The listing builds one solid part. Answer for the finished solid, in the listing's coordinates (mm). A direction names the side the tool comes from. Give positions to 0.01 mm unless a question says otherwise; leave off trailing zeros. Loops run counter-clockwise (first coordinate to the right, second up) from the corner with the lowest first, then second, coordinate; pieces in that order, holes last. Notation, with made-up numbers: (8.5, -18) - (13.5, -18) arc R21 cw to (13.5, -1) - close; hole circle Ø11 at (20, 82). An arc over 180 degrees is marked (long way). Answer as CSV lines item,"result". Start each with the question number.
1) A cutting plane is placed at D-D (z = -90.5). Determine the outline of the cut face in (x, y).
2) Flat-ended cylindrical pins translate along their axes: pin 1 (21 mm diameter, centred on x = -50.5, z = -56, fed in from +Y); pin 2 (1 mm diameter, centred on x = -27.5, z = -137, fed in from +Y). Find the tip coordinate at first contact, or state that the pin passes through.
3) For faces 1 (the face through (-50, 6, -26.65)), 2 (the face through (-49, 4, -65.65)), 3 (the face through (-3, 16, -162)), determine the directions among +Z, -Z, +X, -X, +Y, -Y from which every point of the face is accessible in a straight line to the end or side of a thin tool.
4) Find the intervals of material crossed by line 1 along X through (y, z) = (5.5, -114); line 2 along Z through (x, y) = (-57, 3.5); line 3 along X through (y, z) = (1.75, -34.5), in increasing order.
5) For a pull along Z with two mould halves and no side action, classify faces 4 (the face through (-48, 5, 0)), 5 (the face through (-92, 16, -3)), 6 (the face through (-70, 4, -111.5)) as pulls with the +Z half, pulls with the -Z half, needs draft (parallel to the pull), parting line crosses it, or undercut.
6) A cutting plane is placed at A-A (z = -40.5). Determine the outline of the cut face in (x, y), and give its area (3 significant figures).
7) A cutting plane is placed at B-B (x = -28.5). Determine the outline of the cut face in (y, z), and give its area (3 significant figures).
8) A cutting plane is placed at C-C (x = -57). Determine the outline of the cut face in (y, z).
Autodesk Inventor part; units mm, degrees
ref_plane "YZ Plane" through (0, 0, 0) normal (1, 0, 0) x (0, 1, 0)
ref_plane "XZ Plane" through (0, 0, 0) normal (0, 1, 0) x (-1, 0, 0)
ref_plane "XY Plane" through (0, 0, 0) normal (0, 0, 1) x (1, 0, 0)
sketch "草圖1" plane through (0, 0, 0) normal (0, 1, 0) x (-1, 0, 0)
  line L0 (0, 0) -> (95, 0)
  line L1 (95, 0) -> (95, -165)
  line L2 (95, -165) -> (0, -165)
  line L3 (0, -165) -> (0, 0)
  dimension "d0" = 95
  dimension "d1" = 165
extrude "擠出1" add sketch "草圖1" along normal blind 5
sketch "草圖2" plane through (0, 5, 0) normal (0, 1, 0) x (1, 0, 0)
  circle A0 centre (-3, 3) radius 1.5
  line L0 (0, 0) -> (0, 165)
  line L1 (-95, 0) -> (0, 0)
  circle A1 centre (-92, 3) radius 1.5
  line L2 (-95, 165) -> (-95, 0)
  circle A2 centre (-92, 162) radius 1.5
  line L3 (0, 165) -> (-95, 165)
  circle A3 centre (-3, 162) radius 1.5
  dimension "d4" = 3
  dimension "d5" = 3
  dimension "d6" = 3
  dimension "d7" = 3
  dimension "d8" = 3
  dimension "d9" = 3
  dimension "d10" = 3
  dimension "d11" = 3
  dimension "d12" = 3
  dimension "d13" = 3
  dimension "d14" = 3
  dimension "d15" = 3
extrude "擠出2" add sketch "草圖2" along normal blind 11 contours A0 | A1 | A2 | A3
sketch "草圖3" plane through (0, 0, 0) normal (0, -1, 0) x (1, 0, 0)
  line L0 (-25, -60.15) -> (-20, -60.15)
  line L1 (-20, -60.15) -> (-20, -35.15)
  line L2 (-20, -35.15) -> (-25, -35.15)
  line L3 (-25, -35.15) -> (-25, -60.15)
  line L4 (-95, 0) -> (0, 0)
  line L5 (0, 0) -> (0, -165)
  line L6 (-73, -65.65) -> (-25, -65.65)
  line L7 (-25, -65.65) -> (-25, -29.65)
  line L8 (-25, -29.65) -> (-73, -29.65)
  line L9 (-73, -29.65) -> (-73, -65.65)
  point P0 (-22.5, -35.15)
  point P1 (-20, -47.65)
  point P2 (-25, -47.65)
  dimension "d18" = 35.15
  dimension "d19" = 20
  dimension "d20" = 5
  dimension "d21" = 25
  dimension "d22" = 48
  dimension "d23" = 36
  dimension "d24" = 0
  dimension "d25" = 29.65
extrude "擠出3" cut sketch "草圖3" against normal blind 6 contours L7 L6 L9 L8 L3
sketch "草圖4" plane through (0, 0, 0) normal (0, -1, 0) x (1, 0, 0)
  line L0 (-85, -81.5) -> (-55, -81.5)
  line L1 (-55, -81.5) -> (-55, -111.5)
  line L2 (-55, -111.5) -> (-85, -111.5)
  line L3 (-85, -111.5) -> (-85, -81.5)
  line L4 (0, -165) -> (-95, -165)
  line L5 (-95, -165) -> (-95, 0)
  point P0 (0, 0)
  point P1 (-85, -96.5)
  dimension "d28" = 30
  dimension "d29" = 30
  dimension "d30" = 83.5
  dimension "d31" = 10
extrude "擠出4" cut sketch "草圖4" against normal blind 6
sketch "草圖5" plane through (0, 5, 0) normal (0, 1, 0) x (1, 0, 0)
  line L0 (-25, 26.65) -> (-76, 26.65)
  line L1 (-76, 26.65) -> (-76, 68.65)
  line L2 (-76, 68.65) -> (-25, 68.65)
  line L3 (-25, 68.65) -> (-25, 26.65)
  line L4 (-25, 29.65) -> (-73, 29.65)
  line L5 (-25, 65.65) -> (-25, 29.65)
  line L6 (-73, 65.65) -> (-25, 65.65)
  line L7 (-73, 29.65) -> (-73, 65.65)
  point P0 (0, 0)
  point P1 (-70, 65.65)
  point P2 (-70, 29.65)
  dimension "d34" = 3
  dimension "d35" = 0
  dimension "d36" = 3
  dimension "d40" = 3
extrude "擠出5" add sketch "草圖5" along normal blind 3 contours L0 L1 L2 L3 L6 L7 L4
sketch "草圖6" plane through (0, 5, 0) normal (0, 1, 0) x (1, 0, 0)
  line L0 (-88, 78.5) -> (-55, 78.5)
  line L1 (-55, 78.5) -> (-55, 114.5)
  line L2 (-55, 114.5) -> (-88, 114.5)
  line L3 (-88, 114.5) -> (-88, 78.5)
  line L4 (-85, 81.5) -> (-85, 111.5)
  line L5 (-55, 81.5) -> (-85, 81.5)
  line L6 (-85, 111.5) -> (-55, 111.5)
  line L7 (-55, 111.5) -> (-55, 81.5)
  point P0 (0, 0)
  dimension "d41" = 3
  dimension "d42" = 3
  dimension "d43" = 3
  dimension "d44" = 0
extrude "擠出6" add sketch "草圖6" along normal blind 3 contours L3 L2 L1 L6 L4 L5 L0
sketch "草圖7" plane through (0, 5, 0) normal (0, 1, 0) x (1, 0, 0)
  line L0 (-95, 0) -> (0, 0)
  line L1 (0, 0) -> (0, 165)
  line L2 (0, 165) -> (-95, 165)
  line L3 (-95, 165) -> (-95, 0)
  line L4 (-95, 165) -> (-95, 0)
  line L5 (0, 165) -> (-95, 165)
  line L6 (0, 0) -> (0, 165)
  line L7 (-95, 0) -> (0, 0)
  line L8 (-90, 5) -> (-5, 5)
  line L9 (-5, 5) -> (-5, 160)
  line L10 (-5, 160) -> (-90, 160)
  line L11 (-90, 160) -> (-90, 5)
  dimension "d47" = 5
  dimension "d48" = 5
  dimension "d49" = 5
  dimension "d50" = 5
extrude "擠出7" add sketch "草圖7" along normal blind 5
Ans:
1,outline,"(-95, 0) - (-85, 0) - (-85, 8) - (-88, 8) - (-88, 5) - (-90, 5) - (-90, 10) - (-95, 10) - close; (-55, 0) - (0, 0) - (0, 10) - (-5, 10) - (-5, 5) - (-55, 5) - close"
2,pin 1,"y = 8"
2,pin 2,"y = 5"
3,face 1,"+Y"
3,face 2,"+Y, -Y"
3,face 3,"+Z, -Z, +X, -X, +Y"
4,line 1,"-95 to -90, -88 to -55, -5 to 0"
4,line 2,"-165 to -111.5, -81.5 to -65.65, -29.65 to 0"
4,line 3,"-95 to -73, -25 to 0"
5,face 4,"pulls with the +Z half"
5,face 5,"needs draft"
5,face 6,"undercut"
6,outline,"(-95, 0) - (-73, 0) - (-73, 8) - (-76, 8) - (-76, 5) - (-90, 5) - (-90, 10) - (-95, 10) - close; (-25, 0) - (0, 0) - (0, 10) - (-5, 10) - (-5, 5) - (-25, 5) - close"
6,area,"294 mm2"
7,outline,"(0, -165) - (10, -165) - (10, -160) - (5, -160) - (5, -68.65) - (8, -68.65) - (8, -65.65) - (0, -65.65) - close; (0, -29.65) - (8, -29.65) - (8, -26.65) - (5, -26.65) - (5, -5) - (10, -5) - (10, 0) - (0, 0) - close"
7,area,"713 mm2"
8,outline,"(0, -165) - (10, -165) - (10, -160) - (5, -160) - (5, -114.5) - (8, -114.5) - (8, -111.5) - (0, -111.5) - close; (0, -81.5) - (8, -81.5) - (8, -78.5) - (5, -78.5) - (5, -68.65) - (8, -68.65) - (8, -65.65) - (0, -65.65) - close; (0, -29.65) - (8, -29.65) - (8, -26.65) - (5, -26.65) - (5, -5) - (10, -5) - (10, 0) - (0, 0) - close"
